```python
from build123d import *

# Parameters (mm, degrees)
F2_R = 4
F3_R = 30
F4_T = -1


with BuildPart() as f1:
    # F0 (on Front) → F1 (revolve)
    with BuildSketch(Plane.XZ):
        Polygon((-12.5, 0), (0, 0), (0, 40), (-3, 40), (-12.5, 16), align=None)
    revolve(axis=Axis((0, 0, 20), (0, 0, -1)))

    # F2
    f2_edges = [f1.edges().sort_by_distance(p)[0] for p in [
        (3, 0, 40),
    ]]
    fillet(f2_edges, radius=F2_R)

    # F3
    f3_edges = [f1.edges().sort_by_distance(p)[0] for p in [
        (12.5, 0, 16),
    ]]
    fillet(f3_edges, radius=F3_R)

    # F4
    f4_openings = [f1.faces().sort_by_distance(p)[0] for p in [
        (0, 0, 0),
    ]]
    offset(amount=F4_T, openings=f4_openings)


solid = f1.part
```
Check sheet for the modelled part. Datum: model origin and axes. Units: mm. A direction names the side the tool comes from. Give positions to 0.01 mm unless a question says otherwise; leave off trailing zeros. Order: outer loops, then holes, each group sorted by start corner. A loop starts at its lowest first (then second) coordinate and runs counter-clockwise, first axis right, second up. Notation, with made-up numbers: M 34.25,65 L 44.25,65 A18 ccw 44.25,69 Z; hole C 29.25,77 d3. An arc over 180 degrees is marked long. Answer in a Markdown table with one row per item. Add a question column.
Q1. Thickness scan on L1, parallel to X at y = 0, z = 8; L2, parallel to X at y = 5.25, z = 3.5. Record the ranges inside material, lowest first.
Q2. Gauge pin test, flat ends, axial feed: pin 1 Ø1.5 at (x, z) = (5.5, 13) entering from +Y; pin 2 Ø4 at (x, z) = (9, 23) entering from +Y; pin 3 Ø1 at (x, z) = (-2, 5.5) entering from -Y; pin 4 Ø3 at (x, z) = (9, 29) entering from +Y. Record the tip position at first contact, or that the pin passes through.
Q3. Access from +Z, -Z, +X, -X, +Y, -Y to the whole of each face (thin tool, end or side, straight path). Record for faces 1 (the cylindrical face through (-10.97, 3.45, 5.07)), 2 (the conical face through (-6.23, 1.96, 31.08)).
Q4. Sectioned sample at A-A, the plane z = 6.5. Record the boundary of the cut face in (x, y), and give its area (3 significant figures).
Q5. Sectioned sample at B-B, the plane z = 25.5. Record the boundary of the cut face in (x, y).
Verdict:
| question | item | result |
|---|---|---|
| 1 | L1 | -12.5 to -11.5, 11.5 to 12.5 |
| 1 | L2 | -11.34 to -10.23, 10.23 to 11.34 |
| 2 | pin 1 | y = 11.44 |
| 2 | pin 2 | y = 7.05 |
| 2 | pin 3 | y = -12.41 |
| 2 | pin 4 | through |
| 3 | face 1 | -Z |
| 3 | face 2 | +Z |
| 4 | outline | C 0,0 d25; hole C 0,0 d23 |
| 4 | area | 75.4 mm² |
| 5 | outline | C 0,0 d17.48; hole C 0,0 d15.33 |
